Answer from the drawing. Dimensions are ordinates in mm from the lowest x, y and z of the part. A direction names the side the tool comes from. Round coordinates to 2 decimals unless told otherwise and drop trailing zeros. Loops run counter-clockwise (first coordinate to the right, second up) from the corner with the lowest first, then second, coordinate; pieces in that order, holes last. Notation, with made-up numbers: M 10.25,-21 L 49.25,-21 A28 ccw 49.25,16 Z; hole C 18.5,32 d6. An arc over 180 degrees is marked long. Answer as CSV lines item,"result".
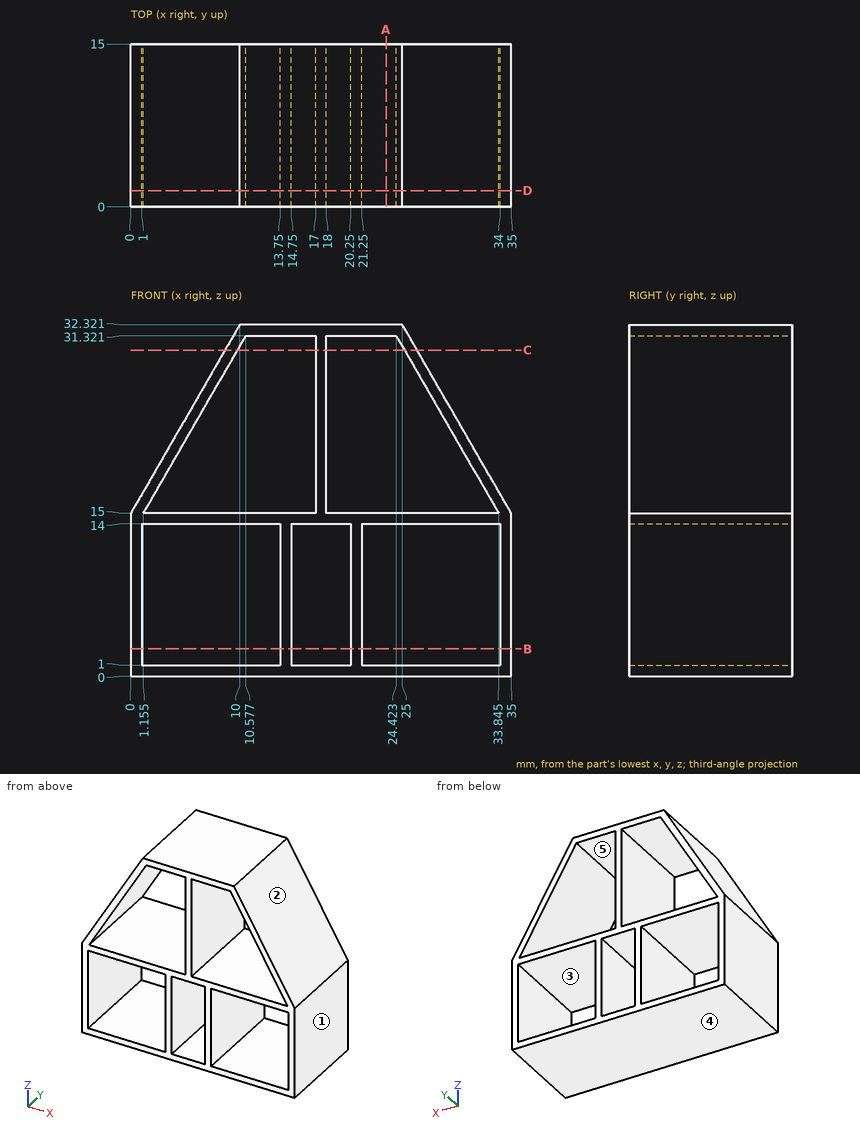
1) Determine the mould class of the marked faces 1, 2 and 3 for opening direction Z: released by +Z, released by -Z, zero draft, split by the parting line, or undercut.
Evaluation:
face 1,"zero draft"
face 2,"released by +Z"
face 3,"undercut"
2) Each of these flat-tipped pins is pushed along its axis until it touches: P1, Ø4, axis at x = 29.5, y = 2.5, coming from the +Z side; P2, Ø3, axis at x = 7, y = 8, coming from the +Z side (1 decimal). Where does it stop, or does it pass through?
Evaluation:
P1,"stops at z = 27.99"
P2,"stops at z = 29.7"
3) Straight lines are drawn through the part: line 1 (X direction, y = 13.25, z = 3.5); line 2 (Z direction, x = 15.5, y = 2.5); line 3 (Z direction, x = 21, y = 4.25). For each, find the intervals that lie inside material, in ascending order.
Evaluation:
line 1,"x = 0 to 1, 13.75 to 14.75, 20.25 to 21.25, 34 to 35"
line 2,"z = 0 to 1, 14 to 15, 31.32 to 32.32"
line 3,"z = 0 to 15, 31.32 to 32.32"
4) Find section D-D, the plane y = 1.5. Count the separate pieces of the cut face and the enclosed holes in it.
Evaluation:
separate pieces,"1"
enclosed holes,"5"
5) Find section A-A, the plane x = 23.5. Give the vertices of the cut face in (y, z).
Evaluation:
outline,"M 0,0 L 15,0 L 15,1 L 0,1 Z; M 0,14 L 15,14 L 15,15 L 0,15 Z; M 0,31.32 L 15,31.32 L 15,32.32 L 0,32.32 Z"
6) Find section C-C, the plane z = 30. Give the vertices of the cut face in (x, y) (1 decimal).
Evaluation:
outline,"M 8.7,0 L 9.8,0 L 9.8,15 L 8.7,15 Z; M 17,0 L 18,0 L 18,15 L 17,15 Z; M 25.2,0 L 26.3,0 L 26.3,15 L 25.2,15 Z"
7) Find section B-B, the plane z = 2.5. Give the vertices of the cut face in (x, y).
Evaluation:
outline,"M 0,0 L 1,0 L 1,15 L 0,15 Z; M 13.75,0 L 14.75,0 L 14.75,15 L 13.75,15 Z; M 20.25,0 L 21.25,0 L 21.25,15 L 20.25,15 Z; M 34,0 L 35,0 L 35,15 L 34,15 Z"
8) A tool of negligible diameter and unlimited length cuts with its end or side. For the marked faces 4 and 5, from which of +Z, -Z, +X, -X, +Y, -Y can it reach the whole face along a straight path? Write none if from no direction.
Evaluation:
face 4,"-Z, +X, -X, +Y, -Y"
face 5,"+Y, -Y"
